Could you check a few things on this model? Use its own coordinates, in mm. Give positions to 0.01 mm unless a question says otherwise; leave off trailing zeros. Order: outer loops, then holes, each group sorted by start corner. A loop starts at its lowest first (then second) coordinate and runs counter-clockwise, first axis right, second up. Notation, with made-up numbers: (20.25, 74.25) -> (33.25, 74.25) arc R18 cw to (33.25, 90.25) -> close; hole circle Ø5 at (88.5, 71). An arc over 180 degrees is marked (long way). One line per item, written item: value.
```python
from build123d import *

# Parameters (mm, degrees)
SKETCH2_R           = 18.0975
BOSS_EXTRUDE1_DEPTH = 24.638
SKETCH3_R           = 2.3368
CUT_EXTRUDE1_DEPTH  = 36.52562535
SKETCH4_R           = 0.7239
BOSS_EXTRUDE2_DEPTH = 1.778


with BuildPart() as part:
    # Sketch2 → Boss-Extrude1 (new body)
    with BuildSketch(Plane(origin=(0, 0, 0), x_dir=(1, 0, 0), z_dir=(0, 1, 0))):
        with Locations(Location((0, 0, 0), (0, 0, 90))):
            Circle(SKETCH2_R)
    extrude(amount=BOSS_EXTRUDE1_DEPTH)

    # Sketch3 → Cut-Extrude1 (cut, through all)
    with BuildSketch(Plane(origin=(0, 24.638, 0), x_dir=(1, 0, 0), z_dir=(0, 1, 0))):
        with Locations(Location((0, 0, 0), (0, 0, 270))):
            Circle(SKETCH3_R)
    extrude(amount=-CUT_EXTRUDE1_DEPTH, mode=Mode.SUBTRACT)

    # Sketch4 → Boss-Extrude2 (add)
    with BuildSketch(Plane.XZ):
        with Locations(Location((15.972995617, 0, 0), (0, 0, 90))):
            Circle(SKETCH4_R)
        with Locations(Location((-16.847197726, 0, 0), (0, 0, 90))):
            Circle(SKETCH4_R)
    extrude(amount=BOSS_EXTRUDE2_DEPTH)

    # Sketch7 → Cut-Revolve1 (revolve, cut)
    with BuildSketch(Plane.XY, mode=Mode.PRIVATE) as cut_revolve1_sk:
        with BuildLine():
            Line((-18.0975, 21.082), (-18.0975, 3.556))
            ThreePointArc((-18.0975, 3.556), (-15.748, 12.319), (-18.0975, 21.082))
        make_face()
    revolve(cut_revolve1_sk.sketch.rotate(Axis((0, 24.735696044, 0), (0, -1, 0)), 90), axis=Axis((0, 24.735696044, 0), (0, -1, 0)), mode=Mode.SUBTRACT)


solid = part.part
```
1) Suppose I cut it at A-A, the plane x = 0. Write out the boundary of the cut face in (y, z), then the cut area to 3 significant figures.
Answer below:
outline: (0, -18.1) -> (3.56, -18.1) arc R17.52 cw to (21.08, -18.1) -> (24.64, -18.1) -> (24.64, -2.34) -> (0, -2.34) -> close; (0, 2.34) -> (24.64, 2.34) -> (24.64, 18.1) -> (21.08, 18.1) arc R17.52 cw to (3.56, 18.1) -> (0, 18.1) -> close
area: 721 mm2
2) We'd pull the mould along X, two halves only. Please class faces 1 (the cylindrical face through (-17.943, 22.835, 2.356)), 2 (the flat face through (4, 24.638, 0)), 3 (the cylindrical face through (16.68, -0.88, -0.16)), 4 (the cylindrical face through (-16.14, -0.88, -0.16)): +X half, -X half, draft (parallel to the pull), parting line (faces both ways), or undercut.
Answer below:
face 1: parting line
face 2: draft
face 3: undercut
face 4: undercut
3) If I drill on line 1 along Y through (x, z) = (-2, -13); line 2 along X through (y, z) = (8.75, 0); line 3 along X through (y, z) = (11.5, 0), over which ranges is the centre line in solid material (lowest first)?
Answer below:
line 1: y = 0 to 24.64
line 2: x = -16.12 to -2.34, 2.34 to 16.12
line 3: x = -15.77 to -2.34, 2.34 to 15.77
4) Suppose I cut it at B-B, the plane z = 0. Write out the boundary of the cut face in (x, y), then the cut area to 3 significant figures.
Answer below:
outline: (-18.1, 0) -> (-17.57, 0) -> (-17.57, -1.78) -> (-16.12, -1.78) -> (-16.12, 0) -> (-2.34, 0) -> (-2.34, 24.64) -> (-18.1, 24.64) -> (-18.1, 21.08) arc R17.52 cw to (-18.1, 3.56) -> close; (2.34, 0) -> (15.25, 0) -> (15.25, -1.78) -> (16.7, -1.78) -> (16.7, 0) -> (18.1, 0) -> (18.1, 3.56) arc R17.52 cw to (18.1, 21.08) -> (18.1, 24.64) -> (2.34, 24.64) -> close
area: 726 mm2
5) For P1, Ø12, axis at y = 9, z = -6.5, coming from the +X side (3 decimals); P2, Ø3, axis at x = 6.5, y = 12, coming from the -Z side; P3, Ø5, axis at y = 20.5, z = -9.5, coming from the +X side, each with a flat end and sliding along its axis, tell me the tip position at first contact or that it passes through.
Answer below:
P1: stops at x = 17.655
P2: stops at z = -14.94
P3: stops at x = 16.66
